Source: CAD feature listing. Evaluate the final solid. Frame: model axes, mm. A direction names the side the tool comes from. Round coordinates to 2 decimals unless told otherwise and drop trailing zeros. Order: outer loops, then holes, each group sorted by start corner. A loop starts at its lowest first (then second) coordinate and runs counter-clockwise, first axis right, second up. Notation, with made-up numbers: (-32.5, 13) - (-0.5, 13) arc R13 cw to (-0.5, 35) - close; hole circle Ø5 at (56.5, -22.5). An arc over 180 degrees is marked (long way). Return JSON: item names as keys, results as strings. Group by question number.
1) Contact query for flat-ended pins moving along their axis: P1, Ø1.3, axis at y = -2.5, z = 4.5, coming from the -X side; P2, Ø10, axis at x = -5, y = 15, coming from the -Z side; P3, Ø10, axis at x = -5, y = 11, coming from the +Z side. Output: stop coordinate, or through.
2) Section A-A, the plane y = 40. Return loops of the section in (x, z) (3 decimals).
3) Mould query, pull axis X, two halves, no side actions, for faces 6 (the flat face through (-10, -2, 2.837)), 7 (the flat face through (-0.144, -1.878, -10.424)), 8 (the flat face through (-10.424, -1.878, 0.144)). Classes: pulls with the +X half, pulls with the -X half, needs draft (parallel to the pull), parting line crosses it, or undercut.
4) Access query for faces 1 (the flat face through (9.492, -2, -4)), 2 (the flat face through (-2.56, -1.88, 10.11)), 3 (the flat face through (7.269, -1.878, -7.472)), 4 (the flat face through (8.363, -1.878, 6.132)), 5 (the flat face through (-4, -2, -9.492)). Directions: +Z, -Z, +X, -X, +Y, -Y. A direction counts if a zero-diameter tool reaches every point of the face in a straight line with its end or side. Return the directions, or none.
5) Section B-B, the plane y = 10.5. Return loops of the section in (x, z) (1 decimal).
6) Ray query, line 1 (Y direction, x = 8, z = -6); line 2 (Z direction, x = 0, y = 33.5); line 3 (Z direction, x = -1, y = 17). Return the intervals inside material, ascending. Write a range as from..to.
```python
from build123d import *

# Parameters (mm, degrees)
F1_DEPTH = 3.81
F2_R     = 1.5875
F3_DEPTH = 37.1983
F4_R     = 0.635
F5_DEPTH = 5.6642


with BuildPart() as f1:
    # F0 (on Front) → F1 (new body)
    with BuildSketch(Plane.XZ):
        Polygon((0.283386, 9.90249), (0, 10.9601), (-2.289223, 9.638416), (-2.836683, 10.586644), (-4.705826, 8.717501), (-5.48005, 9.491725), (-6.801734, 7.202502), (-7.749961, 7.749961), (-8.434115, 5.196664), (-9.491725, 5.48005), (-9.491725, 2.836683), (-10.586644, 2.836683), (-9.90249, 0.283386), (-10.9601, 0), (-9.638416, -2.289223), (-10.586644, -2.836683), (-8.717501, -4.705826), (-9.491725, -5.48005), (-7.202502, -6.801734), (-7.749961, -7.749961), (-5.196664, -8.434115), (-5.48005, -9.491725), (-2.836683, -9.491725), (-2.836683, -10.586644), (-0.283386, -9.90249), (0, -10.9601), (2.289223, -9.638416), (2.836683, -10.586644), (4.705826, -8.717501), (5.48005, -9.491725), (6.801734, -7.202502), (7.749961, -7.749961), (8.434115, -5.196664), (9.491725, -5.48005), (9.491725, -2.836683), (10.586644, -2.836683), (9.90249, -0.283386), (10.9601, 0), (9.638416, 2.289223), (10.586644, 2.836683), (8.717501, 4.705826), (9.491725, 5.48005), (7.202502, 6.801734), (7.749961, 7.749961), (5.196664, 8.434115), (5.48005, 9.491725), (2.836683, 9.491725), (2.836683, 10.586644), align=None)
    extrude(amount=F1_DEPTH)

    # F2 (on Front) → F3 (join)
    with BuildSketch(Plane.XZ):
        Circle(F2_R)
    extrude(amount=-F3_DEPTH)

    # F4 (on face) → F5 (join)
    with BuildSketch(Plane(origin=(0, 37.1983, 0), x_dir=(-1, 0, 0), z_dir=(0, 1, 0))):
        Circle(F4_R)
    extrude(amount=F5_DEPTH)


solid = f1.part
```
Geometry check:
{
 "1": {"P1": "x = -9.49", "P2": "z = -1.59", "P3": "z = 1.59"},
 "2": {"outline": "circle Ø1.27 at (0, 0)"},
 "3": {"face 6": "needs draft", "face 7": "undercut", "face 8": "pulls with the -X half"},
 "4": {"face 1": "-Z, +X, +Y, -Y", "face 2": "+Z, +Y, -Y", "face 3": "-Z, +Y, -Y", "face 4": "+X, +Y, -Y", "face 5": "-Z, -X, +Y, -Y"},
 "5": {"outline": "circle Ø3.2 at (0, 0)"},
 "6": {"line 1": "-3.81..0", "line 2": "-1.59..1.59", "line 3": "-1.23..1.23"}
}
